from build123d import *

# Parameters (mm, degrees)
SKETCH1_R           = 1.5
BOSS_EXTRUDE1_DEPTH = 3.175


with BuildPart() as part:
    # Sketch1 → Boss-Extrude1 (new body)
    with BuildSketch(Plane(origin=(0, 0, 0), x_dir=(1, 0, 0), z_dir=(0, 1, 0))):
        Polygon((0, 7.5), (0, 0), (444.5, 0), (444.5, 15), (0, 15), align=None)
        with Locations(Location((2.5, 2.5, 0), (0, 0, 270))):
            Circle(SKETCH1_R, mode=Mode.SUBTRACT)
        with Locations(Location((12.5, 2.5, 0), (0, 0, 270))):
            Circle(SKETCH1_R, mode=Mode.SUBTRACT)
        with Locations(Location((139.9, 2.5, 0), (0, 0, 270))):
            Circle(SKETCH1_R, mode=Mode.SUBTRACT)
        with Locations(Location((149.9, 2.5, 0), (0, 0, 270))):
            Circle(SKETCH1_R, mode=Mode.SUBTRACT)
        with Locations(Location((2.5, 12.5, 0), (0, 0, 270))):
            Circle(SKETCH1_R, mode=Mode.SUBTRACT)
        with Locations(Location((12.5, 12.5, 0), (0, 0, 270))):
            Circle(SKETCH1_R, mode=Mode.SUBTRACT)
        with Locations(Location((139.9, 12.5, 0), (0, 0, 270))):
            Circle(SKETCH1_R, mode=Mode.SUBTRACT)
        with Locations(Location((149.9, 12.5, 0), (0, 0, 270))):
            Circle(SKETCH1_R, mode=Mode.SUBTRACT)
        with Locations(Location((442, 12.5, 0), (0, 0, 270))):
            Circle(SKETCH1_R, mode=Mode.SUBTRACT)
        with Locations(Location((294.6, 2.5, 0), (0, 0, 270))):
            Circle(SKETCH1_R, mode=Mode.SUBTRACT)
        with Locations(Location((304.6, 2.5, 0), (0, 0, 270))):
            Circle(SKETCH1_R, mode=Mode.SUBTRACT)
        with Locations(Location((432, 2.5, 0), (0, 0, 270))):
            Circle(SKETCH1_R, mode=Mode.SUBTRACT)
        with Locations(Location((442, 2.5, 0), (0, 0, 270))):
            Circle(SKETCH1_R, mode=Mode.SUBTRACT)
        with Locations(Location((294.6, 12.5, 0), (0, 0, 270))):
            Circle(SKETCH1_R, mode=Mode.SUBTRACT)
        with Locations(Location((304.6, 12.5, 0), (0, 0, 270))):
            Circle(SKETCH1_R, mode=Mode.SUBTRACT)
        with Locations(Location((432, 12.5, 0), (0, 0, 270))):
            Circle(SKETCH1_R, mode=Mode.SUBTRACT)
    extrude(amount=BOSS_EXTRUDE1_DEPTH)


solid = part.part
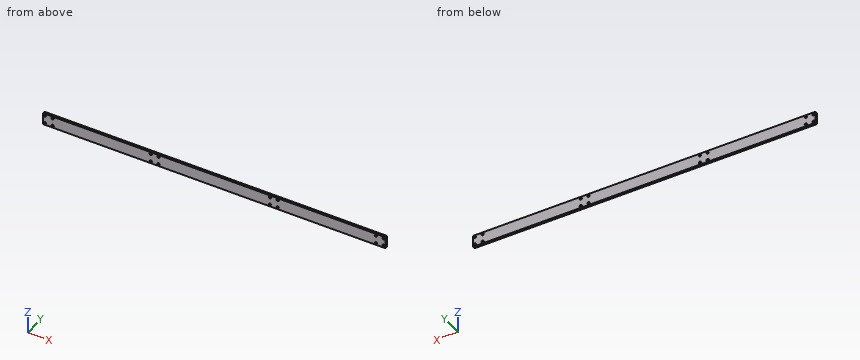
Work out the finished part from the listing and answer in its coordinate system (mm). Give positions to 0.01 mm unless a question says otherwise; leave off trailing zeros. Use a Markdown table: item, result. Add a question column.
1) Consider line 1 along Z through (x, y) = (149.9, 2.35). Determine where the line is inside the solid, lowest interval first.
2) The part is cut by section A-A, the plane y = 2.3. Count the separate pieces of the cut face and the enclosed holes in it, plus the area to 3 significant figures.
3) This flat-tipped pin is pushed along its axis until it touches: P1, Ø1.8, axis at x = 2.5, z = -2.5, coming from the +Y side. Where does it stop, or does it pass through?
Reported:
| question | item | result |
|---|---|---|
| 1 | line 1 | z = -15 to -14, -11 to -4, -1 to 0 |
| 2 | separate pieces | 1 |
| 2 | enclosed holes | 16 |
| 2 | area | 6,550 mm^2 |
| 3 | P1 | passes through |
